Autodesk Inventor part; units mm, degrees
ref_plane "YZ Plane" through (0, 0, 0) normal (1, 0, 0) x (0, 1, 0)
ref_plane "XZ Plane" through (0, 0, 0) normal (0, 1, 0) x (-1, 0, 0)
ref_plane "XY Plane" through (0, 0, 0) normal (0, 0, 1) x (1, 0, 0)
sketch "Sketch1" plane through (0, 0, 0) normal (0, 1, 0) x (-1, 0, 0)
  line L0 (0, 0) -> (20, 0)
  line L1 (20, 0) -> (20, -3)
  line L2 (20, -3) -> (0, -3)
  line L3 (0, -3) -> (0, 0)
  line L4 (0, 0) -> (3, 0)
  line L5 (3, 0) -> (3, -20)
  line L6 (3, -20) -> (0, -20)
  line L7 (0, -20) -> (0, 0)
  dimension "d0" = 3
  dimension "d1" = 3
  dimension "d2" = 20
  dimension "d3" = 20
extrude "Extrusion1" add sketch "Sketch1" along normal blind 165
fillet "Fillet1" radius 2 1 edges at (-3, 82.5, -3)
fillet "Fillet2" radius 5 1 edges at (0, 82.5, 0)
sketch "Sketch2" plane through (-3, 0, -20) normal (-1, 0, 0) x (0, 0, 1)
  line L0 (0, 165) -> (15, 165)
  line L1 (0, 0) -> (15, 0)
  line L2 (0, 0) -> (0, 165)
  point P0 (20, 0)
  point P1 (7.5, 157.5)
  point P2 (7.5, 7.5)
  dimension "d8" = 7.5
  dimension "d9" = 7.5
  dimension "d10" = 150
  dimension "d11" = 7.5
hole "Hole1" at (-3, 157.5, -12.5) at (-3, 7.5, -12.5) direction (1, 0, 0) diameter 4.5 end through all
sketch "Sketch3" plane through (-20, 0, -3) normal (0, 0, -1) x (-1, 0, 0)
  line L0 (-15, 165) -> (0, 165)
  line L1 (-15, 0) -> (0, 0)
  line L2 (0, 0) -> (0, 165)
  point P0 (-20, 0)
  point P1 (-7.5, 157.5)
  point P2 (-7.5, 7.5)
  dimension "d19" = 7.5
  dimension "d20" = 7.5
  dimension "d21" = 7.5
  dimension "d29" = 150
hole "Hole2" at (-12.5, 157.5, -3) at (-12.5, 7.5, -3) direction (0, 0, 1) diameter 4.5 end through all
equation "\"d1\" = d0"
equation "\"d3\" = d2"
properties part number "Top_Angle Bracket" material "Aluminum 6061"
Geometry: final body of the model. Coordinates: model frame, mm. A direction names the side the tool comes from. Give positions to 0.01 mm unless a question says otherwise; leave off trailing zeros. Order: outer loops, then holes, each group sorted by start corner. A loop starts at its lowest first (then second) coordinate and runs counter-clockwise, first axis right, second up. Notation, with made-up numbers: (42.25, 64.5) -> (51.25, 64.5) arc R10 ccw to (51.25, 73.5) -> close; hole circle Ø11 at (83, 2). An arc over 180 degrees is marked (long way). Write each question's results on one line, items separated by ' | '.
1) Cut plane C-C (x = -12.5). Output: boundary loops of the cut face in (y, z).
Geometry says:
outline: (0, -3) -> (5.25, -3) -> (5.25, 0) -> (0, 0) -> close; (9.75, -3) -> (155.25, -3) -> (155.25, 0) -> (9.75, 0) -> close; (159.75, -3) -> (165, -3) -> (165, 0) -> (159.75, 0) -> close
2) Line query: line 1 along Y through (x, z) = (-1.85, -12.5); line 2 along X through (y, z) = (71.5, -16). Output: solid intervals per line, ascending.
Geometry says:
line 1: y = 0 to 5.25, 9.75 to 155.25, 159.75 to 165 | line 2: x = -3 to 0
3) Draft query along Y for faces 1 (the face through (-1.48, 5.98, -14.16)), 2 (the face through (-2.5, 0, -7)), 3 (the face through (-2, 84, -1)). Return one class per face: released by +Y, released by -Y, zero draft, split by the parting line, or undercut.
Geometry says:
face 1: undercut | face 2: released by -Y | face 3: zero draft
4) Cut plane D-D (y = 108). Output: boundary loops of the cut face in (x, z).
Geometry says:
outline: (-20, -3) -> (-5, -3) arc R2 cw to (-3, -5) -> (-3, -20) -> (0, -20) -> (0, -5) arc R5 ccw to (-5, 0) -> (-20, 0) -> close
5) First-contact query: pin 1 Ø12 at (x, y) = (-12.5, 97.5) entering from -Z; pin 2 Ø7.5 at (y, z) = (73, -11) entering from -X. Flat tips, straight axial feed; report the tip coordinate or a pass-through.
Geometry says:
pin 1: stops at z = -3 | pin 2: stops at x = -3
6) Cut plane B-B (z = -12.5). Output: boundary loops of the cut face in (x, y).
Geometry says:
outline: (-3, 0) -> (0, 0) -> (0, 5.25) -> (-3, 5.25) -> close; (-3, 9.75) -> (0, 9.75) -> (0, 155.25) -> (-3, 155.25) -> close; (-3, 159.75) -> (0, 159.75) -> (0, 165) -> (-3, 165) -> close
7) Set-up query: faces 4 (the face through (-13, 81, -3)), 5 (the face through (-14.73, 7.21, -1.48)). Return all of +Z, -Z, +X, -X, +Y, -Y with unobstructed straight access to the full face (end or side cutting, diameter ignored); none if empty.
Geometry says:
face 4: -Z, -X, +Y, -Y | face 5: +Z, -Z
8) Cut plane A-A (y = 7.5). Output: boundary loops of the cut face in (x, z), and give its area (3 significant figures).
Geometry says:
outline: (-20, -3) -> (-14.75, -3) -> (-14.75, 0) -> (-20, 0) -> close; (-10.25, -3) -> (-5, -3) arc R2 cw to (-3, -5) -> (-3, -10.25) -> (0, -10.25) -> (0, -5) arc R5 ccw to (-5, 0) -> (-10.25, 0) -> close; (-3, -20) -> (0, -20) -> (0, -14.75) -> (-3, -14.75) -> close | area: 79.5 mm²
